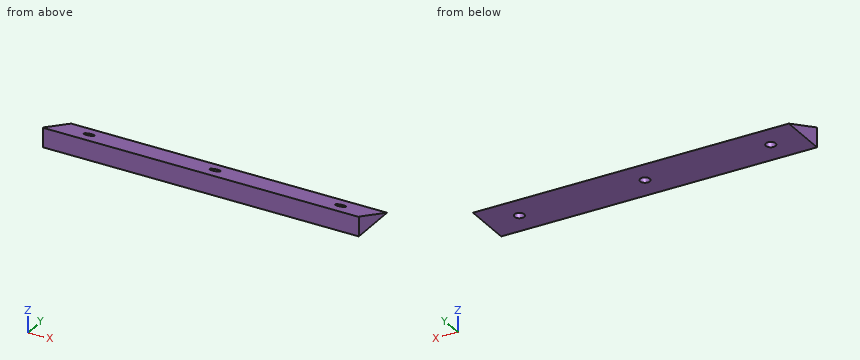
```python
from build123d import *

# Parameters (mm, degrees)
ESBO_O1_W                = 98
ESBO_O1_H                = 25
RESSALTO_EXTRUS_O1_DEPTH = 6
CHANFRO1_SIZE            = 10
CHANFRO1_SIZE_2          = 24.750868534
ESBO_O3_R                = 1.5
CORTE_EXTRUS_O1_DEPTH    = 6


with BuildPart() as part:
    # Esboço1 → Ressalto-extrusão1 (new body)
    with BuildSketch(Plane.XY):
        with Locations((49, -12.5)):
            Rectangle(ESBO_O1_W, ESBO_O1_H)
    extrude(amount=RESSALTO_EXTRUS_O1_DEPTH)

    # Chanfro1
    # the kernel refuses this chamfer: 24.750868534, 10 mm, written as the material it takes off along each edge
    with BuildSketch(Plane(origin=(-64.178729721, 0, 6), x_dir=(0, 0.0881670647319357, -0.9961057015681392), z_dir=(1, 0, 0))) as chanfro1_piece_1:
        Polygon((CHANFRO1_SIZE * 0.996105701568, -CHANFRO1_SIZE * 0.0881670647319), (-CHANFRO1_SIZE_2 * 0.0881670647325, -CHANFRO1_SIZE_2 * 0.996105701575), (0, 0), align=None)
    extrude(amount=226.357459443, mode=Mode.SUBTRACT)

    # Esboço3 → Corte-extrusão1 (cut)
    with BuildSketch(Plane(origin=(0, 0, 0), x_dir=(-1, 0, 0), z_dir=(0, 0, -1))):
        with Locations((-49, -17.5)):
            Circle(ESBO_O3_R)
        with Locations((-10, -17.5)):
            Circle(ESBO_O3_R)
        with Locations((-88, -17.5)):
            Circle(ESBO_O3_R)
    extrude(amount=-CORTE_EXTRUS_O1_DEPTH, mode=Mode.SUBTRACT)


solid = part.part
```
Model file for the job. Use its own axes, mm. Round coordinates to 2 decimals unless told otherwise and drop trailing zeros. Write each loop counter-clockwise with the first axis right and the second up, starting at its lowest first coordinate (ties: lowest second). Pieces come first, ordered by that corner, then holes. Notation, with made-up numbers: M 28,16.5 L 67,16.5 A31 cw 67,45.5 Z; hole C -22,-26 d11. An arc over 180 degrees is marked long. Put each result on its own line as item: value.
Item 1: Cut at C-C (z = 1.45). List the corners of the cut face in (x, y), and give its area (3 significant figures).
Responses:
outline: M 0,-25 L 98,-25 L 98,-13.49 L 0,-13.49 Z; hole C 10,-17.5 d3; hole C 49,-17.5 d3; hole C 88,-17.5 d3
area: 1,110 mm²
Item 2: Cut at A-A (y = -17.5). List the corners of the cut face in (x, z).
Responses:
outline: M 0,0 L 8.5,0 L 8.5,3.07 L 0,3.07 Z; M 11.5,0 L 47.5,0 L 47.5,3.07 L 11.5,3.07 Z; M 50.5,0 L 86.5,0 L 86.5,3.07 L 50.5,3.07 Z; M 89.5,0 L 98,0 L 98,3.07 L 89.5,3.07 Z
Item 3: Probe L1, parallel to X at y = -17.5, z = 1.1; L2, parallel to X at y = -18.5, z = 0.55; L3, parallel to Z at x = 60, y = -19. List the from-to ranges inside material, lowest first. Write a range as from..to.
Responses:
L1: 0..8.5, 11.5..47.5, 50.5..86.5, 89.5..98
L2: 0..8.88, 11.12..47.88, 50.12..86.88, 89.12..98
L3: 0..3.68
Item 4: Cut at D-D (x = 37). List the corners of the cut face in (y, z).
Responses:
outline: M -25,0 L -9.9,0 L -24.75,6 L -25,6 Z
Item 5: Flat gauge pins, fed straight in: P1, Ø3, axis at x = 74.5, y = -21.5, coming from the +Z side; P2, Ø1.5, axis at x = 22, z = 3, coming from the +Y side; P3, Ø2.5, axis at x = 49, y = -17.5, coming from the -Z side; P4, Ø4, axis at x = 88, y = -17.5, coming from the -Z side. Where does each tip first touch, or does it go through?
Responses:
P1: z = 5.29
P2: y = -15.47
P3: through
P4: z = 0
Item 6: Cut at B-B (x = 10). List the corners of the cut face in (y, z), and give its area (3 significant figures).
Responses:
outline: M -25,0 L -19,0 L -19,3.68 L -24.75,6 L -25,6 Z; M -16,0 L -9.9,0 L -16,2.46 Z
area: 36.8 mm²
